Verification items for the finished model (mm, model axes). Coordinates: 2 decimals unless noted, no trailing zeros. Loops run counter-clockwise (first coordinate to the right, second up) from the corner with the lowest first, then second, coordinate; pieces in that order, holes last. Notation, with made-up numbers: (6, 54.5) -> (40, 54.5) arc R36 ccw to (40, 90.5) -> close; hole circle Ø9 at (16.25, 13). An arc over 180 degrees is marked (long way). Answer as a JSON object with one key per item and string values. Group by question number.
Q1. Cross-section at A-A on y = 0.15. Give the number of separate pieces and of enclosed holes in the cut face, and give its area (3 significant figures).
Q2. Release check for a two-part mould opening along X. For faces 1 (the cylindrical face through (0.86, 0.51, 0.9)), 2 (the cylindrical face through (37.2, 0.5, 56.1)), 3 (the cylindrical face through (2.03, 0.51, 19.99)), 4 (the cylindrical face through (36.41, 0.51, 35.62)) record: released by +X, released by -X, zero draft, split by the parting line, or undercut.
Q3. Cross-section at B-B on z = 34.76. Record the boundary of the cut face in (x, y).
Q4. Scan lines: L1, parallel to X at y = 0.65, z = 53.02; L2, parallel to Z at x = 36, y = 0.8; L3, parallel to X at y = 0.3, z = 36. Record each from-to range of solid material in increasing order.
```python
from build123d import *

# Parameters (mm, degrees)
SKETCH2_W           = 38.06
SKETCH2_H           = 57
SKETCH2_R           = 1.53
BOSS_EXTRUDE1_DEPTH = 1
FILLET2_R           = 3
SKETCH4_R           = 1.6
CUT_EXTRUDE1_DEPTH  = 69.54606918


with BuildPart() as part:
    # Sketch2 → Boss-Extrude1 (new body)
    with BuildSketch(Plane(origin=(0, 0, 0), x_dir=(1, 0, 0), z_dir=(0, 1, 0))):
        with Locations((19.03, -28.5)):
            Rectangle(SKETCH2_W, SKETCH2_H)
        with Locations(Location((3, -3, 0), (0, 0, 270))):
            Circle(SKETCH2_R, mode=Mode.SUBTRACT)
        with Locations(Location((3, -21.26, 0), (0, 0, 270))):
            Circle(SKETCH2_R, mode=Mode.SUBTRACT)
        with Locations(Location((3, -34.76, 0), (0, 0, 270))):
            Circle(SKETCH2_R, mode=Mode.SUBTRACT)
        with Locations(Location((3, -53.02, 0), (0, 0, 270))):
            Circle(SKETCH2_R, mode=Mode.SUBTRACT)
        with Locations(Location((35.06, -53.02, 0), (0, 0, 270))):
            Circle(SKETCH2_R, mode=Mode.SUBTRACT)
        with Locations(Location((35.06, -34.76, 0), (0, 0, 270))):
            Circle(SKETCH2_R, mode=Mode.SUBTRACT)
        with Locations(Location((35.06, -21.26, 0), (0, 0, 270))):
            Circle(SKETCH2_R, mode=Mode.SUBTRACT)
        with Locations(Location((35.06, -3, 0), (0, 0, 270))):
            Circle(SKETCH2_R, mode=Mode.SUBTRACT)
    extrude(amount=BOSS_EXTRUDE1_DEPTH)

    # Fillet2
    fillet2_edges = [part.edges().sort_by_distance(p)[0] for p in [
        (38.06, 0.5, 57),
        (0, 0.5, 57),
        (0, 0.5, 0),
        (38.06, 0.5, 0),
    ]]
    fillet(fillet2_edges, radius=FILLET2_R)

    # Sketch4 → Cut-Extrude1 (cut, through all)
    with BuildSketch(Plane(origin=(0, 1, 0), x_dir=(1, 0, 0), z_dir=(0, 1, 0))):
        with Locations(Location((3, -3, 0), (0, 0, 270))):
            Circle(SKETCH4_R)
        with Locations(Location((3, -21.26, 0), (0, 0, 270))):
            Circle(SKETCH4_R)
        with Locations(Location((35.06, -3, 0), (0, 0, 270))):
            Circle(SKETCH4_R)
        with Locations(Location((35.06, -21.26, 0), (0, 0, 270))):
            Circle(SKETCH4_R)
        with Locations(Location((3, -34.76, 0), (0, 0, 270))):
            Circle(SKETCH4_R)
        with Locations(Location((35.06, -34.76, 0), (0, 0, 270))):
            Circle(SKETCH4_R)
        with Locations(Location((3, -53.02, 0), (0, 0, 270))):
            Circle(SKETCH4_R)
        with Locations(Location((35.06, -53.02, 0), (0, 0, 270))):
            Circle(SKETCH4_R)
    extrude(amount=-CUT_EXTRUDE1_DEPTH, mode=Mode.SUBTRACT)


solid = part.part
```
Computed values:
{
 "1": {"separate pieces": "1", "enclosed holes": "8", "area": "2,100 mm²"},
 "2": {"face 1": "released by -X", "face 2": "released by +X", "face 3": "undercut", "face 4": "undercut"},
 "3": {"outline": "(0, 0) -> (1.4, 0) -> (1.4, 1) -> (0, 1) -> close; (4.6, 0) -> (33.46, 0) -> (33.46, 1) -> (4.6, 1) -> close; (36.66, 0) -> (38.06, 0) -> (38.06, 1) -> (36.66, 1) -> close"},
 "4": {"L1": "x = 0 to 1.4, 4.6 to 33.46, 36.66 to 38.06", "L2": "z = 0.15 to 1.71, 4.29 to 19.97, 22.55 to 33.47, 36.05 to 51.73, 54.31 to 56.85", "L3": "x = 0 to 1.99, 4.01 to 34.05, 36.07 to 38.06"}
}
